from build123d import *

# Parameters (mm, degrees)
SKETCH_1_R          = 4.2
SKETCH_1_R_2        = 3
EXTRUDE_1_DEPTH     = 13.5
CUT_EXTRUDE_START   = -1
SKETCH_3_R          = 4.2
CUT_EXTRUDE_3_DEPTH = 1
SKETCH_4_R          = 1
CUT_EXTRUDE_4_DEPTH = 50
MOVE_FACE_1_BY      = 3.5


with BuildPart() as part:
    # ｽｹｯﾁ1 → ﾎﾞｽ - 押し出し1 (new body)
    with BuildSketch(Plane(origin=(0, 0, 0), x_dir=(1, 0, 0), z_dir=(0, 1, 0))):
        with Locations(Location((0, 0, 0), (0, 0, 270))):
            Circle(SKETCH_1_R)
        with Locations(Location((0, 0, 0), (0, 0, 270))):
            Circle(SKETCH_1_R_2, mode=Mode.SUBTRACT)
    extrude(amount=EXTRUDE_1_DEPTH)

    # ｽｹｯﾁ3 → ｶｯﾄ - 押し出し3 (cut)
    with BuildSketch(Plane(origin=(0, 13.5, 0), x_dir=(1, 0, 0), z_dir=(0, 1, 0)).offset(CUT_EXTRUDE_START)):
        with Locations(Location((0, 0, 0), (0, 0, 270))):
            Circle(SKETCH_3_R)
    extrude(amount=CUT_EXTRUDE_3_DEPTH, mode=Mode.SUBTRACT)

    # ｽｹｯﾁ4 → ｶｯﾄ - 押し出し4 (cut, symmetric)
    with BuildSketch(Plane.XY):
        with Locations((0, 12.5)):
            Circle(SKETCH_4_R)
    extrude(amount=CUT_EXTRUDE_4_DEPTH, both=True, mode=Mode.SUBTRACT)

    # Move Face 1: a face moved inward by 3.5
    extrude(part.faces().sort_by_distance((0, 0, 3.36))[0], amount=MOVE_FACE_1_BY, dir=(0, 1, 0), mode=Mode.SUBTRACT)


solid = part.part
Input: part model. Units: mm. Frame: model coordinates. Give positions to 0.01 mm unless a question says otherwise; leave off trailing zeros. Order: outer loops, then holes, each group sorted by start corner. A loop starts at its lowest first (then second) coordinate and runs counter-clockwise, first axis right, second up.
Q1. Contact query for a flat-ended pin moving along its axis: pin 1 Ø2 at (y, z) = (5, -2) entering from +X. Output: stop coordinate, or through.
Checked values:
pin 1: stops at x = 4.08
Q2. Draft query along Z for faces 1 (the flat face through (-3.3, 12.5, -0.1)), 2 (the cylindrical face through (-1.15, 7.94, 2.77)), 3 (the cylindrical face through (1.262, 7.937, 4.006)). Return one class per face: +Z half, -Z half, draft (parallel to the pull), parting line (faces both ways), or undercut.
Checked values:
face 1: draft
face 2: undercut
face 3: parting line
Q3. Section A-A on x = 0. Output: boundary loops of the cut face in (y, z), and give its area (3 significant figures).
Checked values:
outline: (3.5, -4.2) - (11.5, -4.2) - (11.5, -3) - (3.5, -3) - close; (3.5, 3) - (11.5, 3) - (11.5, 4.2) - (3.5, 4.2) - close
area: 19.2 mm2
Q4. Ray query, probe 1 along Z at (x, y) = (0, 9.25); probe 2 along Z at (x, y) = (1, 5.75). Return the intervals inside material, ascending.
Checked values:
probe 1: z = -4.2 to -3, 3 to 4.2
probe 2: z = -4.08 to -2.83, 2.83 to 4.08
Q5. Section C-C on y = 9.5. Output: boundary loops of the cut face in (x, z), and give its area (3 significant figures).
Checked values:
outline: circle Ø8.4 at (0, 0); hole circle Ø6 at (0, 0)
area: 27.1 mm2
Q6. Section B-B on z = 0. Output: boundary loops of the cut face in (x, y).
Checked values:
outline: (-4.2, 3.5) - (-3, 3.5) - (-3, 12.5) - (-4.2, 12.5) - close; (3, 3.5) - (4.2, 3.5) - (4.2, 12.5) - (3, 12.5) - close
